The model under review builds one solid part; all positions refer to its coordinate system, in mm. A direction names the side the tool comes from. Round coordinates to 2 decimals unless told otherwise and drop trailing zeros. Order: outer loops, then holes, each group sorted by start corner. A loop starts at its lowest first (then second) coordinate and runs counter-clockwise, first axis right, second up. Notation, with made-up numbers: M -14,14 L 4,14 A33 ccw 4,51 Z; hole C -38,44 d3. An arc over 180 degrees is marked long. Answer as a JSON object with one key per item and string values. Group by question number.
1. Clearance check with flat-ended pins moving along their axes: P1, Ø12, axis at x = 10, y = -10, coming from the -Z side; P2, Ø7.5, axis at x = -10.5, y = -9, coming from the +Z side; P3, Ø1.5, axis at x = 2.5, z = 3, coming from the +Y side. State where each tip first meets the part, or that it passes through.
2. Mouldability with a two-part tool opening along Y and no side actions: class faces 4 (the face through (1, -20, 2)), 5 (the face through (-10.759, -13.417, 7.535)), 6 (the face through (10.921, -21.142, 15.845)) as released by +Y, released by -Y, zero draft, split by the parting line, or undercut.
3. Machinability: for faces 1 (the face through (-11.63, -17.32, 15.07)), 2 (the face through (37.24, -12.675, 14.483)), 3 (the face through (24.227, -23.028, 9.99)), which of the approach directions +Z, -Z, +X, -X, +Y, -Y give a long, thin tool a straight path to every point of the face, cutting with its end or side? Answer none if there is none.
4. Add section B-B on y = -10. State the section outline as (x, z) points, and give its area (3 significant figures).
5. Add section D-D on x = -37.5. State the section outline as (y, z) points, and give its area (3 significant figures).
6. Add section A-A on z = 12.5. Give the number of separate pieces and of enclosed holes in the cut face, and give its area (3 significant figures).
7. Add section C-C on x = 10. State the section outline as (y, z) points, and give its area (3 significant figures).
8. To check wall thickness, follow probe 1 along Y at (x, z) = (10, 12); probe 2 along Z at (x, y) = (-27.5, -24) (3 decimals); probe 3 along Z at (x, y) = (37.5, -17). State the ranges of each line that lie inside material, in increasing order. Write a range as [from, to].
```python
from build123d import *

# Parameters (mm, degrees)
F1_DEPTH       = 45
F2_R           = 2
F3_DEPTH       = 25.001
F4_D           = 5
F4_CBORE_D     = 8.25
F4_CBORE_DEPTH = 4
F5_R           = 3.5
F5_R_2         = 4.5
F6_DEPTH       = 20.001
F5_R_3         = 7.5
F7_DEPTH       = 10
F9_D           = 2.5
F9_DEPTH       = 12.4
F9_TIP         = 0.7510757738


with BuildPart() as f1:
    # F0 (on Right) → F1 (new body, symmetric)
    with BuildSketch(Plane.YZ):
        Polygon((-25, 20), (-25, 0), (-20, 0), (-20, 5), (0, 5), (0, 20), align=None)
    extrude(amount=F1_DEPTH, both=True)

    # F2 (on face) → F3 (cut, through all)
    with BuildSketch(Plane.XZ.offset(25)):
        with Locations((-37.5, 12.5)):
            Circle(F2_R)
        with Locations((37.5, 12.5)):
            Circle(F2_R)
    extrude(amount=-F3_DEPTH, mode=Mode.SUBTRACT)

    # F4 (through all)
    with Locations(Plane.XZ.offset(25)):
        with Locations((-27.5, 12.5), (27.5, 12.5)):
            CounterBoreHole(F4_D / 2, F4_CBORE_D / 2, F4_CBORE_DEPTH)

    # F5 (on face) → F6 (cut, through all)
    with BuildSketch(Plane.XY.offset(20)):
        with Locations((-10, -10)):
            Circle(F5_R)
        with Locations((10, -10)):
            Circle(F5_R_2)
    extrude(amount=-F6_DEPTH, mode=Mode.SUBTRACT)

    # F5 (on face) → F7 (cut)
    with BuildSketch(Plane.XY.offset(20)):
        with Locations((-10, -10)):
            Circle(F5_R_3)
        with Locations((-10, -10)):
            Circle(F5_R, mode=Mode.SUBTRACT)
        with Locations((10, -10)):
            Circle(F5_R_3)
        with Locations((10, -10)):
            Circle(F5_R_2, mode=Mode.SUBTRACT)
    extrude(amount=-F7_DEPTH, mode=Mode.SUBTRACT)

    # F9
    with Locations(Plane.XZ.offset(25)):
        with Locations((-10, 15), (10, 15)):
            Hole(F9_D / 2, depth=F9_DEPTH)
            with Locations((0, 0, -(F9_DEPTH + F9_TIP / 2))):  # 118° drill point
                Cone(0, F9_D / 2, F9_TIP, mode=Mode.SUBTRACT)


solid = f1.part
```
Recorded:
{
 "1": {"P1": "stops at z = 5", "P2": "stops at z = 10", "P3": "stops at y = -20"},
 "2": {"face 4": "released by +Y", "face 5": "undercut", "face 6": "zero draft"},
 "3": {"face 1": "+Z", "face 2": "+Y, -Y", "face 3": "-Y"},
 "4": {"outline": "M -45,5 L -13.5,5 L -13.5,10 L -17.5,10 L -17.5,20 L -45,20 Z; M -6.5,5 L 5.5,5 L 5.5,10 L 2.5,10 L 2.5,20 L -2.5,20 L -2.5,10 L -6.5,10 Z; M 14.5,5 L 45,5 L 45,20 L 17.5,20 L 17.5,10 L 14.5,10 Z; hole C -37.5,12.5 d4; hole C -27.5,12.5 d5; hole C 27.5,12.5 d5; hole C 37.5,12.5 d4", "area": "906 mm²"},
 "5": {"outline": "M -25,0 L -20,0 L -20,5 L 0,5 L 0,10.5 L -25,10.5 Z; M -25,14.5 L 0,14.5 L 0,20 L -25,20 Z", "area": "300 mm²"},
 "6": {"separate pieces": "5", "enclosed holes": "2", "area": "1,420 mm²"},
 "7": {"outline": "M -25,0 L -20,0 L -20,5 L -14.5,5 L -14.5,10 L -17.5,10 L -17.5,13.75 L -25,13.75 Z; M -25,16.25 L -17.5,16.25 L -17.5,20 L -25,20 Z; M -5.5,5 L 0,5 L 0,20 L -2.5,20 L -2.5,10 L -5.5,10 Z", "area": "186 mm²"},
 "8": {"probe 1": "y = [-25, -17.5], [-2.5, 0]", "probe 2": "z = [0, 8.375], [16.625, 20]", "probe 3": "z = [5, 10.5], [14.5, 20]"}
}
